CAD build for the part. Positions are in the model's coordinates, mm. A direction names the side the tool comes from. Round coordinates to 2 decimals unless told otherwise and drop trailing zeros. Write each loop counter-clockwise with the first axis right and the second up, starting at its lowest first coordinate (ties: lowest second). Pieces come first, ordered by that corner, then holes. Notation, with made-up numbers: (-28, 73) - (30, 73) arc R20 ccw to (30, 109) - close; hole circle Ø5 at (-38.75, 34.25). An arc over 180 degrees is marked (long way). Use one line per item in the form item = value. Start each with the question number.
Item 1: Band-saw the part on C-C, the plane x = 3. List the corners of the cut face in (y, z), and give its area (3 significant figures).
Item 2: Pin check, flat tips, straight feed: pin 1 (0.9 mm diameter, centred on x = -14.5, z = 2, fed in from +Y); pin 2 (1 mm diameter, centred on x = -10, z = 1, fed in from -Y); pin 3 (0.9 mm diameter, centred on y = 17.5, z = 1.5, fed in from +X). Stop position of each tip, or through.
Item 3: Band-saw the part on D-D, the plane y = -11.75. List the corners of the cut face in (x, z).
Item 4: Band-saw the part on A-A, the plane x = -9. List the corners of the cut face in (y, z).
Item 5: Drill centre lines: L1, parallel to X at y = 20, z = 2.25; L2, parallel to Y at x = 7.65, z = 2.3; L3, parallel to Y at x = -26.05, z = 1.5. Where is each one in solid material? Low to high.
Item 6: Band-saw the part on B-B, the plane y = 3. List the corners of the cut face in (x, z), and give its area (3 significant figures).
Item 7: Tool access for faces 1 (the cylindrical face through (-15.894, -0.319, 1.479)), 2 (the cylindrical face through (-1.624, -15.855, 1.479)), 3 (the flat face through (27.65, -11, 1)): list every direction of +Z, -Z, +X, -X, +Y, -Y with a clear straight run to the whole face (end or side of a thin tool).
from build123d import *

# Parameters (mm, degrees)
F0_R     = 1.6
F0_R_2   = 1.25
F0_R_3   = 1.3
F0_R_4   = 19
F1_DEPTH = 3


# Not quite as in the source:
# - ends of sketch curves that miss each other by under 0.0002 mm in the source are joined


with BuildPart() as f1:
    # F0 (on Top) → F1 (new body)
    with BuildSketch(Plane.XY):
        with BuildLine():
            ThreePointArc((26.65, -15.75), (27.3571067812, -15.4571067812), (27.65, -14.75))
            Line((27.65, -14.75), (27.65, -6.142305))
            ThreePointArc((27.65, -6.142305), (27.7581169954, -5.008411416), (28.0785715533, -3.9153822211))
            ThreePointArc((28.0785715533, -3.9153822211), (29.65, 4.25), (28.0785715, 12.4153821998))
            ThreePointArc((28.0785715, 12.4153821998), (27.7581169954, 13.508411416), (27.65, 14.642305))
            Line((27.65, 14.642305), (27.65, 23.25))
            ThreePointArc((27.65, 23.25), (27.3571067812, 23.9571067812), (26.65, 24.25))
            Line((26.65, 24.25), (16.815151, 24.25))
            ThreePointArc((16.815151, 24.25), (7.65, 26.25), (-1.5151510677, 24.2500001477))
            Line((-1.5151510677, 24.2500001477), (-20.35, 24.25))
            ThreePointArc((-20.35, 24.25), (-24.35, 20.25), (-20.35, 16.25))
            Line((-20.35, 16.25), (-19.325715, 16.25))
            ThreePointArc((-19.325715, 16.25), (-15.0422529035, 13.2818239509), (-13.9967824398, 8.1764238984))
            ThreePointArc((-13.9967824398, 8.1764238984), (-14.2174174888, 6.6616493047), (-14.3321842117, 5.1351990085))
            ThreePointArc((-14.3321842117, 5.1351990085), (-15.9346176497, -0.3896755352), (-19.9242382655, -4.5339435787))
            Line((-19.9242382655, -4.5339435787), (-27.969469, -9.604406))
            ThreePointArc((-27.969469, -9.604406), (-29.2019904282, -10.9107598382), (-29.65, -12.65))
            Line((-29.65, -12.65), (-29.65, -22.65))
            ThreePointArc((-29.65, -22.65), (-27.7892401618, -25.8019904282), (-24.1305313003, -25.6955935236))
            Line((-24.1305313003, -25.6955935236), (-11.282229, -17.598022))
            ThreePointArc((-11.282229, -17.598022), (-8.2138844175, -16.2212589687), (-4.884, -15.75))
            Line((-4.884, -15.75), (-2.742305, -15.75))
            ThreePointArc((-2.742305, -15.75), (-1.608411416, -15.8581169954), (-0.5153822211, -16.1785715533))
            ThreePointArc((-0.5153822211, -16.1785715533), (7.65, -17.75), (15.8153821998, -16.1785715))
            ThreePointArc((15.8153821998, -16.1785715), (16.908411416, -15.8581169954), (18.042305, -15.75))
            Line((18.042305, -15.75), (26.65, -15.75))
        make_face()
        with Locations((-26.05, -22.65)):
            Circle(F0_R, mode=Mode.SUBTRACT)
        with Locations((-26.05, -12.65)):
            Circle(F0_R, mode=Mode.SUBTRACT)
        with Locations((-8.35, -11.75)):
            Circle(F0_R, mode=Mode.SUBTRACT)
        with Locations((23.65, -11.75)):
            Circle(F0_R, mode=Mode.SUBTRACT)
        with Locations((-20.35, 20.25)):
            Circle(F0_R_2, mode=Mode.SUBTRACT)
        with Locations((-14.35, 20.25)):
            Circle(F0_R_2, mode=Mode.SUBTRACT)
        with Locations((-8.35, 20.25)):
            Circle(F0_R_3, mode=Mode.SUBTRACT)
        with Locations((7.65, 4.25)):
            Circle(F0_R_4, mode=Mode.SUBTRACT)
        with Locations((23.65, 20.25)):
            Circle(F0_R_3, mode=Mode.SUBTRACT)
    extrude(amount=F1_DEPTH)


solid = f1.part
Determined:
q1.outline = (-17.25, 0) - (-14.17, 0) - (-14.17, 3) - (-17.25, 3) - close; (22.67, 0) - (25.75, 0) - (25.75, 3) - (22.67, 3) - close
q1.area = 18.5 mm²
q2.pin_1 = 24.25
q2.pin_2 = -17.15
q2.pin_3 = 27.65
q3.outline = (-29.54, 0) - (-27.37, 0) - (-27.37, 3) - (-29.54, 3) - close; (-24.73, 0) - (-9.95, 0) - (-9.95, 3) - (-24.73, 3) - close; (-6.75, 0) - (-2.6, 0) - (-2.6, 3) - (-6.75, 3) - close; (17.9, 0) - (22.05, 0) - (22.05, 3) - (17.9, 3) - close; (25.25, 0) - (27.65, 0) - (27.65, 3) - (25.25, 3) - close
q4.outline = (-16.48, 0) - (-13.21, 0) - (-13.21, 3) - (-16.48, 3) - close; (-10.29, 0) - (-4.9, 0) - (-4.9, 3) - (-10.29, 3) - close; (13.4, 0) - (19.12, 0) - (19.12, 3) - (13.4, 3) - close; (21.38, 0) - (24.25, 0) - (24.25, 3) - (21.38, 3) - close
q5.L1 = -24.34 to -21.57, -19.13 to -15.57, -13.13 to -9.63, -7.07 to -2.98, 18.28 to 22.37, 24.93 to 27.65
q5.L2 = -17.75 to -14.75, 23.25 to 26.25
q5.L3 = -26.25 to -24.25, -21.05 to -14.25, -11.05 to -8.39
q6.outline = (-14.61, 0) - (-11.31, 0) - (-11.31, 3) - (-14.61, 3) - close; (26.61, 0) - (29.61, 0) - (29.61, 3) - (26.61, 3) - close
q6.area = 18.9 mm²
q7.face_1 = +Z, -Z, -X
q7.face_2 = +Z, -Z, -Y
q7.face_3 = +Z, -Z, +X, -Y
